from build123d import *

# Parameters (mm, degrees)
IZIM1_W                              = 50
IZIM1_H                              = 18
IZIM1_R                              = 2.001074691
IZIM1_R_2                            = 2.688724503
Y_KSEKLIK_EKSTR_ZYON1_DEPTH          = 3
M5_HELISARMAL_I_IN_Z_VANA_MATKAB_1_D = 5.2
IZIM4_W                              = 50
IZIM4_H                              = 3
Y_KSEKLIK_EKSTR_ZYON2_DEPTH          = 15
IZIM5_W                              = 50
IZIM5_H                              = 2.5
KES_EKSTR_ZYON1_DEPTH                = 15


with BuildPart() as part:
    # Çizim1 → Yükseklik-Ekstrüzyon1 (new body)
    # profile 1 of 3: a face of its own
    with BuildSketch(Plane.XY):
        with Locations((10.655737705, -2.06557377)):
            Rectangle(IZIM1_W, IZIM1_H)
        with Locations((25.655737705, -1.06557377)):
            Circle(IZIM1_R, mode=Mode.SUBTRACT)
        with Locations((-4.344262295, -1.06557377)):
            Circle(IZIM1_R_2, mode=Mode.SUBTRACT)
    # profile 2 of 3: a face of its own
    with BuildSketch(Plane.XY):
        with Locations((25.655737705, -1.06557377)):
            Circle(IZIM1_R)
    # profile 3 of 3: a face of its own
    with BuildSketch(Plane.XY):
        with Locations((-4.344262295, -1.06557377)):
            Circle(IZIM1_R_2)
    extrude(amount=Y_KSEKLIK_EKSTR_ZYON1_DEPTH)

    # M5 Helisarmal için Zıvana matkabı1 (through all)
    with Locations(Plane(origin=(0, 0, 0), x_dir=(-1, 0, 0), z_dir=(0, 0, -1))):
        with Locations((-25.655737705, -1.06557377), (4.344262295, -1.06557377)):
            Hole(M5_HELISARMAL_I_IN_Z_VANA_MATKAB_1_D / 2)

    # Çizim4 → Yükseklik-Ekstrüzyon2 (add)
    with BuildSketch(Plane.XY.offset(3)):
        with Locations((10.655737705, -9.56557377)):
            Rectangle(IZIM4_W, IZIM4_H)
    extrude(amount=Y_KSEKLIK_EKSTR_ZYON2_DEPTH)

    # Çizim5 → Kes-Ekstrüzyon1 (cut)
    with BuildSketch(Plane.XY.offset(3)):
        with Locations((10.655737705, 5.68442623)):
            Rectangle(IZIM5_W, IZIM5_H)
    extrude(amount=-KES_EKSTR_ZYON1_DEPTH, mode=Mode.SUBTRACT)


solid = part.part
The listing builds one solid part. Answer for the finished solid, in the listing's coordinates (mm). A direction names the side the tool comes from. Round coordinates to 2 decimals unless told otherwise and drop trailing zeros. Order: outer loops, then holes, each group sorted by start corner. A loop starts at its lowest first (then second) coordinate and runs counter-clockwise, first axis right, second up. Notation, with made-up numbers: M 64.25,-1.5 L 93.25,-1.5 A30 cw 93.25,21.5 Z; hole C 14,-25 d5. An arc over 180 degrees is marked long. Answer in a Markdown table with one row per item. Add a question column.
1) The part is cut by section C-C on z = 2. Determine the outline of the cut face in (x, y), plus the area to 3 significant figures.
2) Determine the mould class of faces 1 (the face through (10, -2, 3)), 2 (the face through (-1.864, -0.285, 1.521)), 3 (the face through (35.656, -9, 5)) for opening direction X: pulls with the +X half, pulls with the -X half, needs draft (parallel to the pull), parting line crosses it, or undercut.
3) Consider line 1 along X through (y, z) = (-3, 2.25); line 2 along X through (y, z) = (1.25, 2); line 3 along Z through (x, y) = (19, -6.25). Determine where each line is inside the solid, lowest interval first. Write a range as from..to.
4) The part is cut by section D-D on y = 1. Determine the outline of the cut face in (x, z), plus the area to 3 significant figures.
5) Which of the six approach directions +Z, -Z, +X, -X, +Y, -Y give full straight-line access (tool end or side, diameter ignored) to faces 4 (the face through (23.06, -0.95, 1.52)), 5 (the face through (10, -8.066, 10))?
6) The part is cut by section B-B on x = 25. Determine the outline of the cut face in (y, z).
7) Flat-ended cylindrical pins translate along their axes: pin 1 Ø4 at (x, y) = (25.66, -1.07) entering from -Z; pin 2 Ø8 at (x, z) = (8, 11.5) entering from +Y. Find the tip coordinate at first contact, or state that the pin passes through.
8) The part is cut by section A-A on y = -2.25. Determine the outline of the cut face in (x, z).
Findings below:
| question | item | result |
|---|---|---|
| 1 | outline | M -14.34,-11.07 L 35.66,-11.07 L 35.66,4.43 L -14.34,4.43 Z; hole C -4.34,-1.07 d5.2; hole C 25.66,-1.07 d5.2 |
| 1 | area | 733 mm² |
| 2 | face 1 | needs draft |
| 2 | face 2 | undercut |
| 2 | face 3 | pulls with the +X half |
| 3 | line 1 | x = -14.34..-6.08, -2.61..23.92, 27.39..35.66 |
| 3 | line 2 | x = -14.34..-5.53, -3.16..24.47, 26.84..35.66 |
| 3 | line 3 | z = 0..3 |
| 4 | outline | M -14.34,0 L -5.92,0 L -5.92,3 L -14.34,3 Z; M -2.77,0 L 24.08,0 L 24.08,3 L -2.77,3 Z; M 27.23,0 L 35.66,0 L 35.66,3 L 27.23,3 Z |
| 4 | area | 131 mm² |
| 5 | face 4 | +Z, -Z |
| 5 | face 5 | +Z, +X, -X, +Y |
| 6 | outline | M -11.07,0 L -3.58,0 L -3.58,3 L -8.07,3 L -8.07,18 L -11.07,18 Z; M 1.45,0 L 4.43,0 L 4.43,3 L 1.45,3 Z |
| 7 | pin 1 | passes through |
| 7 | pin 2 | stops at y = -8.07 |
| 8 | outline | M -14.34,0 L -6.66,0 L -6.66,3 L -14.34,3 Z; M -2.03,0 L 23.34,0 L 23.34,3 L -2.03,3 Z; M 27.97,0 L 35.66,0 L 35.66,3 L 27.97,3 Z |
